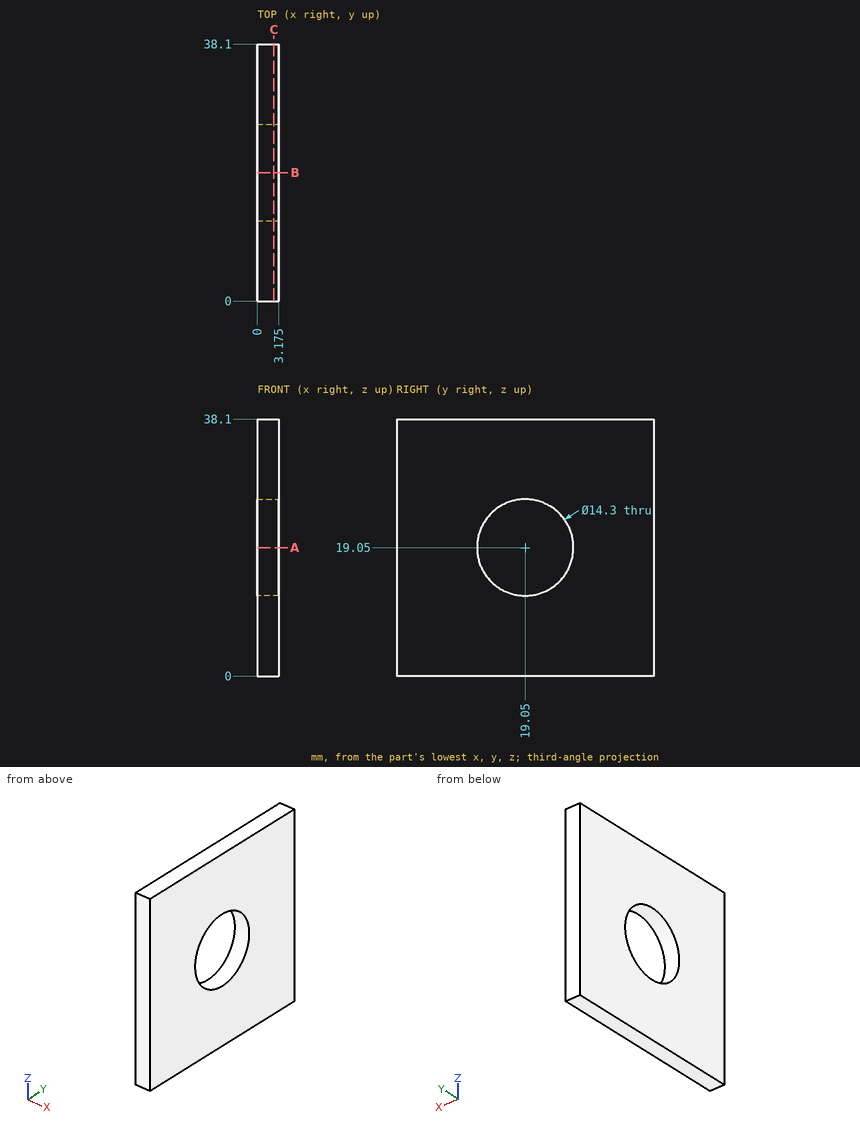
Geometry: see drawing. Coordinates: mm, zero at the bounding-box minimum. Give positions to 0.01 mm unless a question says otherwise; leave off trailing zeros. Loops run counter-clockwise (first coordinate to the right, second up) from the corner with the lowest first, then second, coordinate; pieces in that order, holes last. Notation, with made-up numbers: (28, 23) -> (62, 23) arc R35 ccw to (62, 59) -> close; hole circle Ø2 at (46.5, -15). An arc over 180 degrees is marked (long way). Put each result on its own line as item: value.
1. Cut plane A-A (z = 19.05). Return the cut outline in (x, y) (1 decimal).
Taken from the geometry:
outline: (0, 0) -> (3.2, 0) -> (3.2, 11.9) -> (0, 11.9) -> close; (0, 26.2) -> (3.2, 26.2) -> (3.2, 38.1) -> (0, 38.1) -> close
2. Ray query, line 1 along Y through (x, z) = (1.4, 19.05); line 2 along Y through (x, z) = (0.25, 20.5); line 3 along Z through (x, y) = (2.9, 16.5). Return the intervals inside material, ascending. Write a range as [from, to].
Taken from the geometry:
line 1: y = [0, 11.9], [26.2, 38.1]
line 2: y = [0, 12.05], [26.05, 38.1]
line 3: z = [0, 12.37], [25.73, 38.1]
3. Cut plane C-C (x = 2.45). Return the cut outline in (y, z).
Taken from the geometry:
outline: (0, 0) -> (38.1, 0) -> (38.1, 38.1) -> (0, 38.1) -> close; hole circle Ø14.3 at (19.05, 19.05)
